from build123d import *

# Parameters (mm, degrees)
F1_DEPTH = 25.4
F3_D     = 3.2512
F4_R     = 3.3655
F5_DEPTH = 25.4


with BuildPart() as f1:
    # F0 (on Front) → F1 (new body)
    with BuildSketch(Plane.XZ):
        Polygon((1.5875, 25.4), (0, 25.4), (0, 0), (25.4, 0), (25.4, 1.5875), (1.5875, 1.5875), align=None)
    extrude(amount=F1_DEPTH)

    # F3 (through all)
    with Locations(Plane(origin=(0, 0, 0), x_dir=(0, -1, 0), z_dir=(-1, 0, 0))):
        with Locations((4.1275, 21.082), (21.2725, 7.874)):
            Hole(F3_D / 2)

    # F4 (on face) → F5 (cut)
    with BuildSketch(Plane.XY.offset(1.5875)):
        with Locations((13.49375, -19.05)):
            Circle(F4_R)
        with Locations((13.49375, -6.35)):
            Circle(F4_R)
    extrude(amount=-F5_DEPTH, mode=Mode.SUBTRACT)


solid = f1.part
The listing builds one solid part. Answer for the finished solid, in the listing's coordinates (mm). A direction names the side the tool comes from. Give positions to 0.01 mm unless a question says otherwise; leave off trailing zeros. Loops run counter-clockwise (first coordinate to the right, second up) from the corner with the lowest first, then second, coordinate; pieces in that order, holes last. Notation, with made-up numbers: M 68.25,-23.5 L 96.25,-23.5 A21 ccw 96.25,2.5 Z; hole C -14.5,70 d3. An arc over 180 degrees is marked long. Answer as CSV lines item,"result".
Item 1: The part is cut by section C-C (y = -1.5). Give the vertices of the cut face in (x, z), and give its area (3 significant figures).
Values follow:
outline,"M 0,0 L 25.4,0 L 25.4,1.59 L 1.59,1.59 L 1.59,25.4 L 0,25.4 Z"
area,"78.1 mm^2"
Item 2: Which of the six approach directions +Z, -Z, +X, -X, +Y, -Y give full straight-line access (tool end or side, diameter ignored) to faces 1 (the flat face through (14, -13, 1.588)), 2 (the cylindrical face through (12.764, -22.335, 0.805))?
Values follow:
face 1,"+Z, +X, +Y, -Y"
face 2,"+Z, -Z"
Item 3: A straight line is drawn through the part: line 1 along X through (y, z) = (-22.5, 5.75). Find the intervals that lie inside material, in ascending order. Write a range as [from, to].
Values follow:
line 1,"x = [0, 1.59]"
Item 4: The mould has two halves that part along Y. Classify faces 3 (the cylindrical face through (0.8, -4.5, 19.5)), 4 (the flat face through (1, 0, 7)), 5 (the flat face through (1.588, -13, 13)): released by +Y, released by -Y, zero draft, split by the parting line, or undercut.
Values follow:
face 3,"undercut"
face 4,"released by +Y"
face 5,"zero draft"
Item 5: The part is cut by section A-A (y = -19.05). Give the vertices of the cut face in (x, z), and give its area (3 significant figures).
Values follow:
outline,"M 0,0 L 10.13,0 L 10.13,1.59 L 1.59,1.59 L 1.59,25.4 L 0,25.4 Z; M 16.86,0 L 25.4,0 L 25.4,1.59 L 16.86,1.59 Z"
area,"67.4 mm^2"
Item 6: The part is cut by section B-B (x = 11.75). Give the vertices of the cut face in (y, z).
Values follow:
outline,"M -25.4,0 L -21.93,0 L -21.93,1.59 L -25.4,1.59 Z; M -16.17,0 L -9.23,0 L -9.23,1.59 L -16.17,1.59 Z; M -3.47,0 L 0,0 L 0,1.59 L -3.47,1.59 Z"
Item 7: Given pin 1 Ø2.5 at (y, z) = (-4.13, 21.08) entering from +X; pin 2 Ø6 at (x, y) = (15.5, -17.5) entering from +Z, each flat-ended and moving along its own axis, determine where each tip first touches the part or whether it passes through.
Values follow:
pin 1,"passes through"
pin 2,"stops at z = 1.59"
Item 8: The part is cut by section D-D (z = 11.5). Give the vertices of the cut face in (x, y), and give its area (3 significant figures).
Values follow:
outline,"M 0,-25.4 L 1.59,-25.4 L 1.59,0 L 0,0 Z"
area,"40.3 mm^2"
